Can you work these out from the model? Positions are in its coordinate system, mm. Face numbers are marked on the shaded views. A direction names the side the tool comes from. Round coordinates to 2 decimals unless told otherwise and drop trailing zeros. Write each loop counter-clockwise with the first axis right and the second up, starting at its lowest first coordinate (ties: lowest second). Pieces come first, ordered by that corner, then holes. Notation, with made-up numbers: M 64,6 L 123,6 A20 ccw 123,28 Z; hole C -4,65.25 d7. An arc over 180 degrees is marked long. Use one line per item in the form item = value. Start each with the question number.
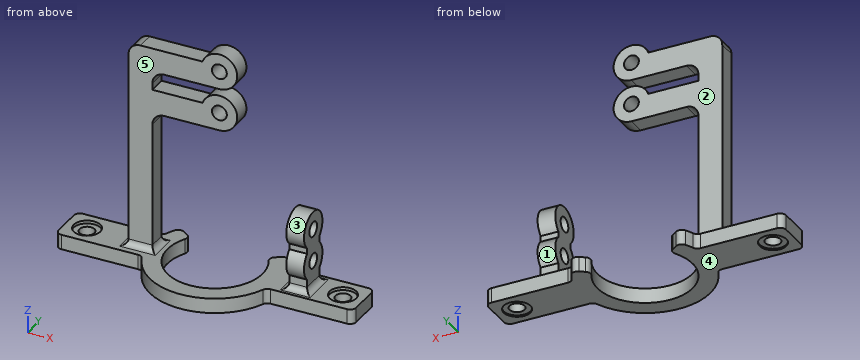
```python
from build123d import *

# Parameters (mm, degrees)
SKETCH1_R                = 2.55
BOSS_EXTRUDE1_DEPTH      = 5
SKETCH4_R                = 4.5
CUT_EXTRUDE2_DEPTH       = 1
SKETCH6_W                = 5.947651005
SKETCH6_H                = 20
BOSS_EXTRUDE2_DEPTH      = 4
BOSS_EXTRUDE2_DEPTH_BACK = 4
SKETCH11_R               = 4.5
CUT_EXTRUDE3_DEPTH       = 0.5
SKETCH16_R               = 2.5
BOSS_EXTRUDE3_DEPTH      = 3
BOSS_EXTRUDE3_DEPTH_BACK = 3
FILLET3_R                = 2
BOSS_EXTRUDE4_DEPTH      = 5.947651
CUT_EXTRUDE5_REACH       = 85
SKETCH18_R               = 2.5


with BuildPart() as part:
    # Sketch1 → Boss-Extrude1 (new body)
    with BuildSketch(Plane.XY):
        with BuildLine():
            Line((100, 25), (100, 20))
            ThreePointArc((100, 20), (99.414213562, 18.585786438), (98, 18))
            Line((98, 18), (72.248595461, 18))
            ThreePointArc((72.248595461, 18), (71.130561473, 17.658312395), (70.39454584, 16.75))
            ThreePointArc((70.39454584, 16.75), (50, 3), (29.60545416, 16.75))
            ThreePointArc((29.60545416, 16.75), (28.869438527, 17.658312395), (27.751404539, 18))
            Line((27.751404539, 18), (2, 18))
            ThreePointArc((2, 18), (0.585786438, 18.585786438), (0, 20))
            Line((0, 20), (0, 25))
            Line((0, 25), (0, 30))
            ThreePointArc((0, 30), (0.585786438, 31.414213562), (2, 32))
            Line((2, 32), (21.056240945, 32))
            Line((21.056240945, 32), (27.751404539, 32))
            ThreePointArc((27.751404539, 32), (28.869438527, 32.341687605), (29.60545416, 33.25))
            ThreePointArc((29.60545416, 33.25), (30.166752838, 34.520625347), (30.807119991, 35.753295167))
            ThreePointArc((30.807119991, 35.753295167), (32.106461975, 36.725482012), (33.699080137, 36.414026968))
            Line((33.699080137, 36.414026968), (35.34656276, 35.260447216))
            ThreePointArc((35.34656276, 35.260447216), (36.146649881, 34.078494315), (35.955031011, 32.664127224))
            ThreePointArc((35.955031011, 32.664127224), (50, 9), (64.044968989, 32.664127224))
            ThreePointArc((64.044968989, 32.664127224), (63.853350119, 34.078494315), (64.65343724, 35.260447216))
            Line((64.65343724, 35.260447216), (66.300919863, 36.414026968))
            ThreePointArc((66.300919863, 36.414026968), (67.893538025, 36.725482012), (69.192880009, 35.753295167))
            ThreePointArc((69.192880009, 35.753295167), (69.833247162, 34.520625347), (70.39454584, 33.25))
            ThreePointArc((70.39454584, 33.25), (71.130561473, 32.341687605), (72.248595461, 32))
            Line((72.248595461, 32), (78.943759055, 32))
            Line((78.943759055, 32), (98, 32))
            ThreePointArc((98, 32), (99.414213562, 31.414213562), (100, 30))
            Line((100, 30), (100, 25))
        make_face()
        with Locations((93, 25)):
            Circle(SKETCH1_R, mode=Mode.SUBTRACT)
        with Locations((7, 25)):
            Circle(SKETCH1_R, mode=Mode.SUBTRACT)
    extrude(amount=BOSS_EXTRUDE1_DEPTH)

    # Sketch4 → Cut-Extrude2 (cut)
    with BuildSketch(Plane.XY.offset(5)):
        with Locations((93, 25)):
            Circle(SKETCH4_R)
        with Locations((7, 25)):
            Circle(SKETCH4_R)
    extrude(amount=-CUT_EXTRUDE2_DEPTH, mode=Mode.SUBTRACT)

    # Sketch6 → Boss-Extrude2 (add, two sides)
    with BuildSketch(Plane(origin=(0, 25, 0), x_dir=(-1, 0, 0), z_dir=(0, -1, 0))) as boss_extrude2_sk:
        with Locations((-80.026174497, -15)):
            Rectangle(SKETCH6_W, SKETCH6_H)
    extrude(amount=BOSS_EXTRUDE2_DEPTH)
    extrude(boss_extrude2_sk.sketch, amount=-BOSS_EXTRUDE2_DEPTH_BACK)

    # Sketch11 → Cut-Extrude3 (cut)
    with BuildSketch(Plane(origin=(0, 0, 0), x_dir=(-1, 0, 0), z_dir=(0, 0, -1))):
        with Locations((-93, 25)):
            Circle(SKETCH11_R)
        with Locations((-7, 25)):
            Circle(SKETCH11_R)
    extrude(amount=-CUT_EXTRUDE3_DEPTH, mode=Mode.SUBTRACT)

    # Sketch16 → Boss-Extrude3 (add, two sides)
    with BuildSketch(Plane(origin=(0, 25, 0), x_dir=(-1, 0, 0), z_dir=(0, -1, 0))) as boss_extrude3_sk:
        with BuildLine():
            Line((-30.494270905, -5), (-22.494270905, -5))
            Line((-22.494270905, -5), (-22.494270905, -71))
            ThreePointArc((-22.494270905, -71), (-23.665843781, -73.828427125), (-26.494270905, -75))
            Line((-26.494270905, -75), (-30.494270905, -75))
            Line((-30.494270905, -75), (-47.361403242, -75))
            ThreePointArc((-47.361403242, -75), (-57.917236977, -76.464101615), (-53.018257491, -67))
            Line((-53.018257491, -67), (-34.494270905, -67))
            ThreePointArc((-34.494270905, -67), (-31.665843781, -65.828427125), (-30.494270905, -63))
            Line((-30.494270905, -63), (-30.494270905, -60.732138804))
            Line((-30.494270905, -60.732138804), (-47.361403242, -60.732138804))
            ThreePointArc((-47.361403242, -60.732138804), (-57.917236977, -62.196240419), (-53.018257491, -52.732138804))
            Line((-53.018257491, -52.732138804), (-34.494270905, -52.732138804))
            ThreePointArc((-34.494270905, -52.732138804), (-31.665843781, -51.560565928), (-30.494270905, -48.732138804))
            Line((-30.494270905, -48.732138804), (-30.494270905, -5))
        make_face()
        with Locations((-53.018257491, -73)):
            Circle(SKETCH16_R, mode=Mode.SUBTRACT)
        with Locations((-53.018257491, -58.732138804)):
            Circle(SKETCH16_R, mode=Mode.SUBTRACT)
    extrude(amount=BOSS_EXTRUDE3_DEPTH)
    extrude(boss_extrude3_sk.sketch, amount=-BOSS_EXTRUDE3_DEPTH_BACK)

    # Fillet3
    fillet3_edges = [part.edges().sort_by_distance(p)[0] for p in [
        (83, 25, 5),
        (80.026174498, 29, 5),
        (77.052348995, 25, 5),
        (80.026174498, 21, 5),
        (30.494270905, 25, 5),
        (26.494270905, 28, 5),
        (22.494270905, 25, 5),
        (26.494270905, 22, 5),
    ]]
    fillet(fillet3_edges, radius=FILLET3_R)

    # Sketch17 → Boss-Extrude4 (add)
    with BuildSketch(Plane(origin=(83, 0, 0), x_dir=(0, 0, -1), z_dir=(1, 0, 0))):
        with BuildLine():
            ThreePointArc((-19.547210182, 27.503414308), (-31, 25), (-19.547210182, 22.496585692))
            ThreePointArc((-19.547210182, 22.496585692), (-8.094420363, 25), (-19.547210182, 27.503414308))
        make_face()
    extrude(amount=-BOSS_EXTRUDE4_DEPTH)

    # Sketch18 → Cut-Extrude5 (cut, up to next)
    with BuildSketch(Plane(origin=(83, 0, 0), x_dir=(0, 0, -1), z_dir=(1, 0, 0)), mode=Mode.PRIVATE) as cut_extrude5_sk1:
        with Locations((-25, 25)):
            Circle(SKETCH18_R)
    cut_extrude5_tool1 = extrude(cut_extrude5_sk1.sketch, amount=-CUT_EXTRUDE5_REACH, mode=Mode.PRIVATE) & part.part
    add(cut_extrude5_tool1.solids().sort_by_distance((83, 25, 25))[0], mode=Mode.SUBTRACT)
    # Sketch18 → Cut-Extrude5 (cut, up to next)
    with BuildSketch(Plane(origin=(83, 0, 0), x_dir=(0, 0, -1), z_dir=(1, 0, 0)), mode=Mode.PRIVATE) as cut_extrude5_sk2:
        with Locations((-14.094420363, 25)):
            Circle(SKETCH18_R)
    cut_extrude5_tool2 = extrude(cut_extrude5_sk2.sketch, amount=-CUT_EXTRUDE5_REACH, mode=Mode.PRIVATE) & part.part
    add(cut_extrude5_tool2.solids().sort_by_distance((83, 25, 14.09442))[0], mode=Mode.SUBTRACT)


solid = part.part
```
1. If we section it at B-B (x = 93): List the corners of the cut face in (y, z) for me, and give its area (4 significant figures).
2. Will these pins go through, and if not, where does the flat tip stop? pin 1 (5 mm diameter, centred on x = 27.5, z = 58.5, fed in from -Y); pin 2 (1.8 mm diameter, centred on y = 24.5, z = 62, fed in from +X); pin 3 (18.5 mm diameter, centred on x = 32, z = 25.5, fed in from +Y).
3. If we section it at C-C (y = 13.5): List the corners of the cut face in (x, z) for me (3 decimals).
4. If we mould it in two halves opening along Z, with no side actions, what happens to the marked faces 3, 4 and 5? For each: pulls with the +Z half, pulls with the -Z half, needs draft (parallel to the pull), parting line crosses it, or undercut.
5. If we section it at D-D (x = 42.5): List the corners of the cut face in (y, z) for me.
6. If we section it at A-A (z = 25): List the corners of the cut face in (x, y) for me.
7. Please list where these lines run through material, in increasing order: line 1 along X through (y, z) = (25, 2.55); line 2 along Z through (x, y) = (52, 23.5); line 3 along Y through (x, z) = (81.75, 25).
8. Which directions (+Z, -Z, +X, -X, +Y, -Y) give clear straight access to the entire face, cutting with the end or side of a thin tool? Please do the marked faces 1 and 2.
Model answer:
q1.outline = M 18,0 L 20.5,0 L 20.5,0.5 L 22.45,0.5 L 22.45,4 L 20.5,4 L 20.5,5 L 18,5 Z; M 27.55,0.5 L 29.5,0.5 L 29.5,0 L 32,0 L 32,5 L 29.5,5 L 29.5,4 L 27.55,4 Z
q1.area = 38.65 mm2
q2.pin_1 = 22
q2.pin_2 = 58.53
q2.pin_3 = 28
q3.outline = M 31.245,0 L 38.876,0 L 38.876,5 L 31.245,5 Z; M 61.124,0 L 68.755,0 L 68.755,5 L 61.124,5 Z
q4.face_3 = undercut
q4.face_4 = pulls with the -Z half
q4.face_5 = needs draft
q5.outline = M 4.32,0 L 10.87,0 L 10.87,5 L 4.32,5 Z; M 22,52.73 L 28,52.73 L 28,60.73 L 22,60.73 Z; M 22,67 L 28,67 L 28,75 L 22,75 Z
q6.outline = M 22.49,22 L 30.49,22 L 30.49,28 L 22.49,28 Z; M 77.05,19 L 83,19 L 83,22.5 L 77.05,22.5 Z; M 77.05,27.5 L 83,27.5 L 83,31 L 77.05,31 Z
q7.line_1 = 0 to 4.45, 9.55 to 34, 66 to 90.45, 95.55 to 100
q7.line_2 = 52.73 to 56.45, 61.02 to 64.65, 67 to 70.72, 75.28 to 78.91
q7.line_3 = 19 to 22.5, 27.5 to 31
q8.face_1 = +X, -X, +Y
q8.face_2 = +Z, -X, +Y
